Geometry: see drawing. Coordinates: mm, zero at the bounding-box minimum. A direction names the side the tool comes from. Coordinates: 2 decimals unless noted, no trailing zeros. Order: outer loops, then holes, each group sorted by start corner. A loop starts at its lowest first (then second) coordinate and runs counter-clockwise, first axis right, second up.
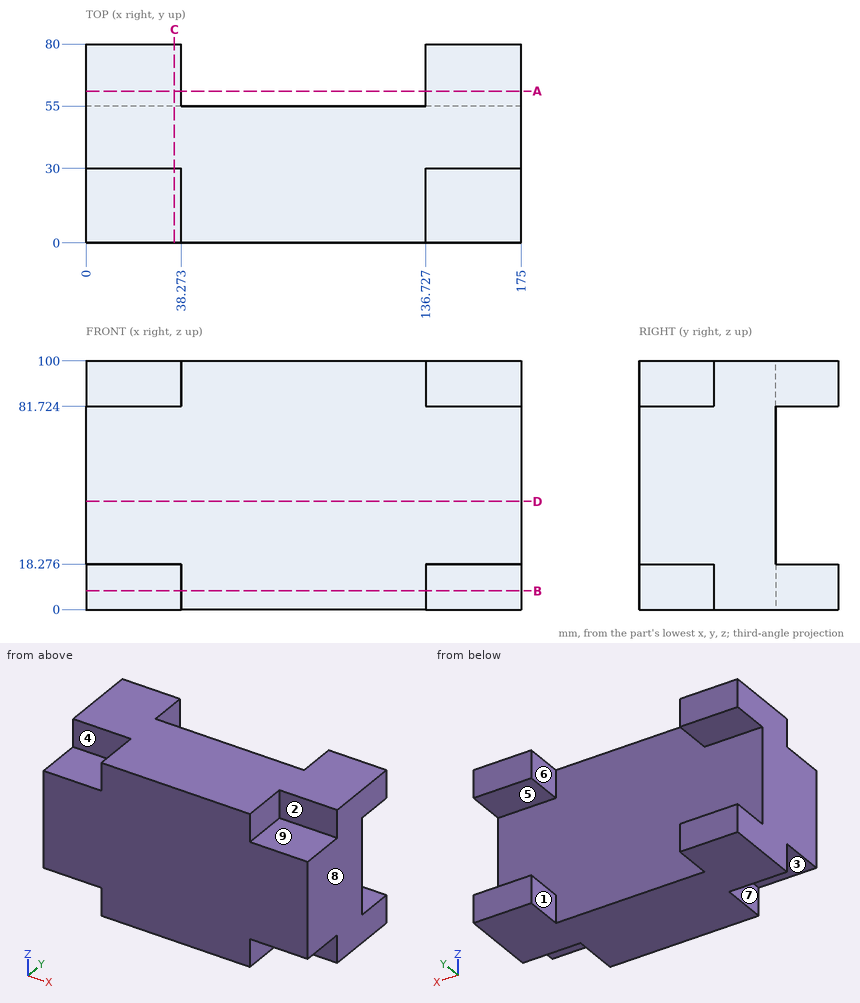
Q1. Section query C-C on x = 35.5. Output: boundary loops of the cut face in (y, z), plus the area to 3 significant figures.
Solutions:
outline: (0, 18.28) - (30, 18.28) - (30, 0) - (80, 0) - (80, 18.28) - (55, 18.28) - (55, 81.72) - (80, 81.72) - (80, 100) - (30, 100) - (30, 81.72) - (0, 81.72) - close
area: 5,320 mm2
Q2. Section query A-A on y = 61. Output: boundary loops of the cut face in (x, z).
Solutions:
outline: (0, 0) - (38.27, 0) - (38.27, 18.28) - (0, 18.28) - close; (0, 81.72) - (38.27, 81.72) - (38.27, 100) - (0, 100) - close; (136.73, 0) - (175, 0) - (175, 18.28) - (136.73, 18.28) - close; (136.73, 81.72) - (175, 81.72) - (175, 100) - (136.73, 100) - close
Q3. Pull-direction query (X, two-part tool) for the marked faces 6, 7, 8 and 9; classes: pulls with the +X half, pulls with the -X half, needs draft (parallel to the pull), parting line crosses it, or undercut.
Solutions:
face 6: undercut
face 7: pulls with the -X half
face 8: pulls with the +X half
face 9: needs draft
Q4. Section query B-B on z = 7.5. Output: boundary loops of the cut face in (x, y), plus the area to 3 significant figures.
Solutions:
outline: (0, 30) - (38.27, 30) - (38.27, 0) - (136.73, 0) - (136.73, 30) - (175, 30) - (175, 80) - (136.73, 80) - (136.73, 55) - (38.27, 55) - (38.27, 80) - (0, 80) - close
area: 9,240 mm2
Q5. Material intervals for line 1 along Z through (x, y) = (160, 71); line 2 along Y through (x, z) = (8.5, 94); line 3 along Y through (x, z) = (161, 65), sorted ascending.
Solutions:
line 1: z = 0 to 18.28, 81.72 to 100
line 2: y = 30 to 80
line 3: y = 0 to 55
Q6. Section query D-D on z = 43.5. Output: boundary loops of the cut face in (x, y), plus the area to 4 significant figures.
Solutions:
outline: (0, 0) - (175, 0) - (175, 55) - (0, 55) - close
area: 9,625 mm2
Q7. Set-up query: the marked faces 1, 2, 3, 4 and 5. Return all of +Z, -Z, +X, -X, +Y, -Y with unobstructed straight access to the full face (end or side cutting, diameter ignored); none if empty.
Solutions:
face 1: +Z, -Z, +Y
face 2: +Z, +X, -Y
face 3: -Z, -X, -Y
face 4: +Z, -X, -Y
face 5: +X, -X, +Y
Q8. Pin query (flat end, axial travel): P1, Ø2, axis at y = 69, z = 13, coming from the -X side; P2, Ø14.5, axis at y = 8, z = 95, coming from the -X side; P3, Ø15, axis at x = 153.5, y = 16.5, coming from the +Z side; P4, Ø5.5, axis at x = 154, z = 93, coming from the -Y side. Return the tip coordinate at first contact, or that it passes through.
Solutions:
P1: stops at x = 0
P2: stops at x = 38.27
P3: stops at z = 81.72
P4: stops at y = 30
